from build123d import *

# Parameters (mm, degrees)
SKETCH1_W                        = 250
SKETCH1_H                        = 175
BOSS_EXTRUDE1_DEPTH              = 120
SKETCH3_W                        = 250
SKETCH3_H                        = 75
CUT_EXTRUDE1_DEPTH               = 25
CUT_EXTRUDE2_REACH               = 329.91
SKETCH4_W                        = 20
SKETCH4_H                        = 30
F_20_0MM_DOWEL_HOLE1_D           = 20
F_20_0MM_DOWEL_HOLE1_CSINK_D     = 20.05
F_20_0MM_DOWEL_HOLE1_CSINK_ANGLE = 90
F_20_0MM_DOWEL_HOLE2_D           = 20
F_20_0MM_DOWEL_HOLE2_CSINK_D     = 20.05
F_20_0MM_DOWEL_HOLE2_CSINK_ANGLE = 90
CUT_EXTRUDE3_REACH               = 329.91
CUT_EXTRUDE4_REACH               = 329.91


with BuildPart() as part:
    # Sketch1 → Boss-Extrude1 (new body)
    with BuildSketch(Plane(origin=(0, 0, 0), x_dir=(1, 0, 0), z_dir=(0, 1, 0))):
        with Locations((125, 87.5)):
            Rectangle(SKETCH1_W, SKETCH1_H)
    extrude(amount=BOSS_EXTRUDE1_DEPTH)

    # Sketch3 → Cut-Extrude1 (cut)
    with BuildSketch(Plane(origin=(0, 120, 0), x_dir=(1, 0, 0), z_dir=(0, 1, 0))):
        with Locations((125, 87.5)):
            Rectangle(SKETCH3_W, SKETCH3_H)
    extrude(amount=-CUT_EXTRUDE1_DEPTH, mode=Mode.SUBTRACT)

    # Sketch4 → Cut-Extrude2 (cut, up to next)
    with BuildSketch(Plane.XY, mode=Mode.PRIVATE) as cut_extrude2_sk1:
        with Locations((10, 50)):
            Rectangle(SKETCH4_W, SKETCH4_H)
    cut_extrude2_tool1 = extrude(cut_extrude2_sk1.sketch, amount=-CUT_EXTRUDE2_REACH, mode=Mode.PRIVATE) & part.part
    add(cut_extrude2_tool1.solids().sort_by_distance((10, 50, 0))[0], mode=Mode.SUBTRACT)

    # Ø20.0mm Dowel Hole1 (through all)
    with Locations(Plane.XY):
        with Locations((50, 25)):
            CounterSinkHole(F_20_0MM_DOWEL_HOLE1_D / 2, F_20_0MM_DOWEL_HOLE1_CSINK_D / 2, counter_sink_angle=F_20_0MM_DOWEL_HOLE1_CSINK_ANGLE)

    # Ø20.0mm Dowel Hole2 (through all)
    with Locations(Plane(origin=(0, 120, 0), x_dir=(1, 0, 0), z_dir=(0, 1, 0))):
        with Locations((40, 150)):
            CounterSinkHole(F_20_0MM_DOWEL_HOLE2_D / 2, F_20_0MM_DOWEL_HOLE2_CSINK_D / 2, counter_sink_angle=F_20_0MM_DOWEL_HOLE2_CSINK_ANGLE)

    # Sketch11 → Cut-Extrude3 (cut, up to next)
    with BuildSketch(Plane.XY, mode=Mode.PRIVATE) as cut_extrude3_sk1:
        Polygon((90, 120), (250, 27.62395693), (250, 120), align=None)
    cut_extrude3_tool1 = extrude(cut_extrude3_sk1.sketch, amount=-CUT_EXTRUDE3_REACH, mode=Mode.PRIVATE) & part.part
    add(cut_extrude3_tool1.solids().sort_by_distance((196.666667, 89.207986, 0))[0], mode=Mode.SUBTRACT)

    # Sketch12 → Cut-Extrude4 (cut, up to next)
    with BuildSketch(Plane(origin=(0, 120, 0), x_dir=(1, 0, 0), z_dir=(0, 1, 0)), mode=Mode.PRIVATE) as cut_extrude4_sk1:
        Polygon((75, 0), (250, 101.036297108), (250, 0), align=None)
    cut_extrude4_tool1 = extrude(cut_extrude4_sk1.sketch, amount=-CUT_EXTRUDE4_REACH, mode=Mode.PRIVATE) & part.part
    add(cut_extrude4_tool1.solids().sort_by_distance((191.666667, 120, -33.678766))[0], mode=Mode.SUBTRACT)


solid = part.part
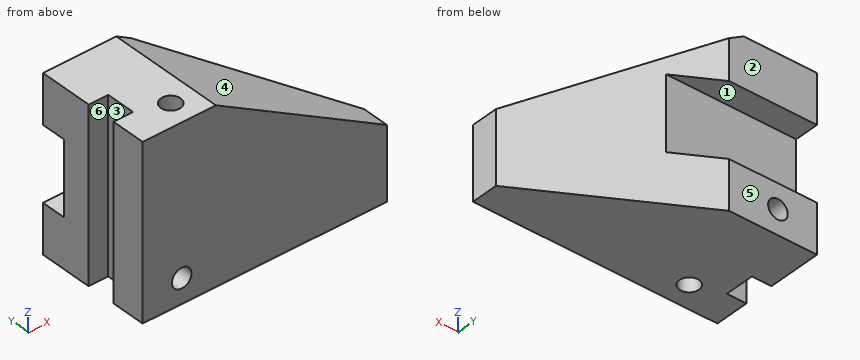
Could you check a few things on this model? Use its own coordinates, in mm. Face numbers are marked on the shaded views. A direction names the side the tool comes from. Coordinates: 2 decimals unless noted, no trailing zeros. Order: outer loops, then holes, each group sorted by start corner. A loop starts at its lowest first (then second) coordinate and runs counter-clockwise, first axis right, second up.
Q1. Will these pins go through, and if not, where does the flat tip stop? pin 1 (24 mm diameter, centred on y = 52, z = -63.5, fed in from -X); pin 2 (12 mm diameter, centred on x = 40, z = -150, fed in from +Y); pin 3 (7.5 mm diameter, centred on x = 92, y = 108.5, fed in from +Z); pin 4 (16 mm diameter, centred on x = 7, z = -63.5, fed in from +Y).
Q2. Thinking about a two-plate mould opening in Y: for the marked faces 4, 5 and 6, which applies, released by +Y, released by -Y, zero draft, split by the parting line, or undercut?
Q3. Suppose I cut it at A-A on z = -150. Please give me the cut outline in (x, y) (3 decimals).
Q4. Which directions (+Z, -Z, +X, -X, +Y, -Y) give clear straight access to the entire face, cutting with the end or side of a thin tool? Please do the marked faces 1, 2 and 3.
Q5. Suppose I cut it at C-C on z = -112.5. Please give me the cut outline in (x, y).
Q6. Suppose I cut it at B-B on y = 25. Please give me the cut outline in (x, z) (3 decimals), and give its area (3 significant figures).
Q7. Please list where these lines run through material, in increasing order: L1, parallel to Y at x = 50, z = -58.5; L2, parallel to X at y = 24.5, z = -121; L3, parallel to Z at x = 40, y = 55.5.
Q8. Suppose I cut it at D-D on y = 7. Please give me the cut outline in (x, z).
Answer:
1. pin 1: stops at x = 20
1. pin 2: passes through
1. pin 3: stops at z = -7.65
1. pin 4: stops at y = 95
2. face 4: zero draft
2. face 5: released by +Y
2. face 6: undercut
3. outline: (0, 0) - (30, 0) - (30, 119.975) - (29.975, 120) - (0, 120) - (0, 65) - (20, 65) - (20, 35) - (0, 35) - close; (50, 0) - (250, 0) - (250, 27.624) - (90, 120) - (50.025, 120) - (50, 119.975) - (50, 35) arc R10 cw to (50, 15) - close
4. face 1: +X, -X, +Y
4. face 2: +Z, -Z, +X, -X, +Y
4. face 3: +Z, -Z, -X
5. outline: (0, 0) - (250, 0) - (250, 27.62) - (133.3, 95) - (0, 95) - (0, 65) - (20, 65) - (20, 35) - (0, 35) - close; hole circle Ø20 at (50, 25)
6. outline: (0, -175) - (40, -175) - (40, -160) arc R10 cw to (40, -140) - (40, -0.025) - (39.975, 0) - (0, 0) - close; (60, -175) - (250, -175) - (250, -101.036) - (75, 0) - (60.025, 0) - (60, -0.025) - close
6. area: 31,300 mm2
7. L1: y = 0 to 15, 35 to 95
7. L2: x = 0 to 40.01, 59.99 to 250
7. L3: z = -175 to -160, -140 to 0
8. outline: (0, -175) - (250, -175) - (250, -101.04) - (75, 0) - (0, 0) - close; hole circle Ø20 at (40, -150)
